```python
from build123d import *

# Parameters (mm, degrees)
SKETCH_1_R          = 7.65
EXTRUDE_1_DEPTH     = 3
SKETCH_2_R          = 5
CUT_EXTRUDE_1_DEPTH = 366.286189172
FILLET_1_R          = 20
SKETCH_3_R          = 1.65
CUT_EXTRUDE_2_DEPTH = 366.286189172
FILLET_2_R          = 40
FILLET_3_R          = 80
SKETCH_4_W          = 105
SKETCH_4_H          = 60
CUT_EXTRUDE_3_DEPTH = 366.286189172
FILLET_4_R          = 5
CUT_EXTRUDE_4_DEPTH = 269.344927286
FILLET_5_R          = 2
FILLET_6_R          = 8
EXTRUDE_START       = -3
EXTRUDE_2_DEPTH     = 3
SKETCH_7_R          = 1.65
CUT_EXTRUDE_5_DEPTH = 3


with BuildPart() as part:
    # 草图1 → 凸台-拉伸1 (new body)
    with BuildSketch(Plane.XY):
        with BuildLine():
            Line((106.954174428, -60), (20.632339437, 21.778580517))
            ThreePointArc((20.632339437, 21.778580517), (-21.778580517, 20.632339437), (-20.632339437, -21.778580517))
            Line((-20.632339437, -21.778580517), (83.045825572, -120))
            Line((83.045825572, -120), (345, -120))
            Line((345, -120), (345, -60))
            Line((345, -60), (106.954174428, -60))
        make_face()
        Circle(SKETCH_1_R, mode=Mode.SUBTRACT)
    extrude(amount=EXTRUDE_1_DEPTH)

    # 草图2 → 切除-拉伸1 (cut, through all)
    with BuildSketch(Plane.XY.offset(3)):
        with Locations((305, -90)):
            Circle(SKETCH_2_R)
        with Locations((278, -90)):
            Circle(SKETCH_2_R)
        with Locations((332, -90)):
            Circle(SKETCH_2_R)
    extrude(amount=-CUT_EXTRUDE_1_DEPTH, mode=Mode.SUBTRACT)

    # 圆角1
    fillet_1_edges = [part.edges().sort_by_distance(p)[0] for p in [
        (345, -60, 1.5),
        (345, -120, 1.5),
    ]]
    fillet(fillet_1_edges, radius=FILLET_1_R)

    # 草图3 → 切除-拉伸2 (cut, through all)
    with BuildSketch(Plane.XY.offset(3)):
        with Locations((216.4, -115.5)):
            Circle(SKETCH_3_R)
        with Locations((216.5, -64.5)):
            Circle(SKETCH_3_R)
        with Locations((191.5, -64.5)):
            Circle(SKETCH_3_R)
        with Locations((191.4, -115.5)):
            Circle(SKETCH_3_R)
        with Locations((14.114048497, -48.497460089)):
            Circle(SKETCH_3_R)
        with Locations((49.18902554, -11.473873209)):
            Circle(SKETCH_3_R)
        with Locations((67.385880926, -28.616640024)):
            Circle(SKETCH_3_R)
        with Locations((32.310903883, -65.640226903)):
            Circle(SKETCH_3_R)
        with BuildLine():
            Line((222.8, -113.85), (235, -113.85))
            ThreePointArc((235, -113.85), (236.65, -115.5), (235, -117.15))
            Line((235, -117.15), (222.8, -117.15))
            ThreePointArc((222.8, -117.15), (221.15, -115.5), (222.8, -113.85))
        make_face()
        with BuildLine():
            Line((222.8, -66.15), (235, -66.15))
            ThreePointArc((235, -66.15), (236.65, -64.5), (235, -62.85))
            Line((235, -62.85), (222.8, -62.85))
            ThreePointArc((222.8, -62.85), (221.15, -64.5), (222.8, -66.15))
        make_face()
        with BuildLine():
            Line((36.821084288, 2.51599917), (45.677707032, -5.874485534))
            ThreePointArc((45.677707032, -5.874485534), (45.740750291, -8.207086132), (43.408149694, -8.270129391))
            Line((43.408149694, -8.270129391), (34.55152695, 0.120355313))
            ThreePointArc((34.55152695, 0.120355313), (34.488483691, 2.452955911), (36.821084288, 2.51599917))
        make_face()
        with BuildLine():
            Line((19.942962631, -51.650354523), (28.799585375, -60.040839228))
            ThreePointArc((28.799585375, -60.040839228), (28.862628634, -62.373439825), (26.530028037, -62.436483085))
            Line((26.530028037, -62.436483085), (17.673405293, -54.04599838))
            ThreePointArc((17.673405293, -54.04599838), (17.610362034, -51.713397783), (19.942962631, -51.650354523))
        make_face()
        with BuildLine():
            Line((197.8, -113.85), (210, -113.85))
            ThreePointArc((210, -113.85), (211.65, -115.5), (210, -117.15))
            Line((210, -117.15), (197.8, -117.15))
            ThreePointArc((197.8, -117.15), (196.15, -115.5), (197.8, -113.85))
        make_face()
        with BuildLine():
            Line((197.8, -66.15), (210, -66.15))
            ThreePointArc((210, -66.15), (211.65, -64.5), (210, -62.85))
            Line((210, -62.85), (197.8, -62.85))
            ThreePointArc((197.8, -62.85), (196.15, -64.5), (197.8, -66.15))
        make_face()
        with BuildLine():
            Line((172.8, -113.85), (185, -113.85))
            ThreePointArc((185, -113.85), (186.65, -115.5), (185, -117.15))
            Line((185, -117.15), (172.8, -117.15))
            ThreePointArc((172.8, -117.15), (171.15, -115.5), (172.8, -113.85))
        make_face()
        with BuildLine():
            Line((172.8, -66.15), (185, -66.15))
            ThreePointArc((185, -66.15), (186.65, -64.5), (185, -62.85))
            Line((185, -62.85), (172.8, -62.85))
            ThreePointArc((172.8, -62.85), (171.15, -64.5), (172.8, -66.15))
        make_face()
        with BuildLine():
            Line((1.746107245, -34.507587709), (10.602729989, -42.898072413))
            ThreePointArc((10.602729989, -42.898072413), (10.665773248, -45.230673011), (8.333172651, -45.29371627))
            Line((8.333172651, -45.29371627), (-0.523450093, -36.903231566))
            ThreePointArc((-0.523450093, -36.903231566), (-0.586493353, -34.570630968), (1.746107245, -34.507587709))
        make_face()
        with BuildLine():
            Line((55.017939675, -14.626767644), (63.874562418, -23.017252349))
            ThreePointArc((63.874562418, -23.017252349), (63.937605678, -25.349852946), (61.60500508, -25.412896206))
            Line((61.60500508, -25.412896206), (52.748382337, -17.022411501))
            ThreePointArc((52.748382337, -17.022411501), (52.685339077, -14.689810904), (55.017939675, -14.626767644))
        make_face()
        with BuildLine():
            Line((38.139818017, -68.793121338), (46.996440761, -77.183606042))
            ThreePointArc((46.996440761, -77.183606042), (47.05948402, -79.51620664), (44.726883423, -79.579249899))
            Line((44.726883423, -79.579249899), (35.870260679, -71.188765195))
            ThreePointArc((35.870260679, -71.188765195), (35.80721742, -68.856164597), (38.139818017, -68.793121338))
        make_face()
        with BuildLine():
            Line((73.214795061, -31.769534459), (82.071417805, -40.160019163))
            ThreePointArc((82.071417805, -40.160019163), (82.134461064, -42.492619761), (79.801860466, -42.55566302))
            Line((79.801860466, -42.55566302), (70.945237723, -34.165178315))
            ThreePointArc((70.945237723, -34.165178315), (70.882194463, -31.832577718), (73.214795061, -31.769534459))
        make_face()
    extrude(amount=-CUT_EXTRUDE_2_DEPTH, mode=Mode.SUBTRACT)

    # 圆角2
    fillet_2_edges = [part.edges().sort_by_distance(p)[0] for p in [
        (106.954174428, -60, 1.5),
    ]]
    fillet(fillet_2_edges, radius=FILLET_2_R)

    # 圆角3
    fillet_3_edges = [part.edges().sort_by_distance(p)[0] for p in [
        (83.045825572, -120, 1.5),
    ]]
    fillet(fillet_3_edges, radius=FILLET_3_R)

    # 草图4 → 切除-拉伸3 (cut, through all)
    with BuildSketch(Plane.XY.offset(3)):
        with Locations((292.5, -90)):
            Rectangle(SKETCH_4_W, SKETCH_4_H)
    extrude(amount=-CUT_EXTRUDE_3_DEPTH, mode=Mode.SUBTRACT)

    # 圆角4
    fillet_4_edges = [part.edges().sort_by_distance(p)[0] for p in [
        (240, -120, 1.5),
        (240, -60, 1.5),
    ]]
    fillet(fillet_4_edges, radius=FILLET_4_R)

    # 草图5 → 切除-拉伸4 (cut, through all)
    with BuildSketch(Plane.XY.offset(3)):
        Polygon((170.8, -107.073879127), (170.8, -72.926120873), (196.643481613, -90), align=None)
        Polygon((107.673788457, -69), (162.8, -69), (162.8, -112), align=None)
        Polygon((182.624652559, -71.15), (203.9, -85.205873586), (225.175347441, -71.15), align=None)
        Polygon((211.156518387, -90), (237, -72.926120873), (237, -107.073879127), align=None)
        Polygon((182.624652559, -108.85), (203.9, -94.794126414), (225.175347441, -108.85), align=None)
        Polygon((104.589547434, -76.740160666), (149.792834925, -112), (90.539471777, -112), align=None)
        Polygon((83.107750181, -109.038663458), (97.619712786, -72.619680215), (53.254218477, -80.756370264), align=None)
        Polygon((60.248478543, -73.373540194), (82.827238337, -49.540404857), (100.242066861, -66.038663458), align=None)
        Polygon((12.415001138, -37.631100304), (37.481546744, -42.016378913), (43.304983555, -66.895294173), align=None)
        Polygon((38.334111759, -10.557272346), (44.066420967, -35.046871816), (68.740714664, -39.36352773), align=None)
        Polygon((46.048599826, -43.515146043), (73.041613266, -48.237451473), (52.282913666, -70.149412161), align=None)
    extrude(amount=-CUT_EXTRUDE_4_DEPTH, mode=Mode.SUBTRACT)

    # 圆角5
    fillet_5_edges = [part.edges().sort_by_distance(p)[0] for p in [
        (53.254218477, -80.756370264, 1.5),
        (97.619712786, -72.619680215, 1.5),
        (104.589547434, -76.740160666, 1.5),
        (149.792834925, -112, 1.5),
        (100.242066861, -66.038663458, 1.5),
        (60.248478543, -73.373540194, 1.5),
        (82.827238337, -49.540404857, 1.5),
        (43.304983555, -66.895294173, 1.5),
        (12.415001138, -37.631100304, 1.5),
        (37.481546744, -42.016378913, 1.5),
        (237, -107.073879127, 1.5),
        (211.156518387, -90, 1.5),
        (237, -72.926120873, 1.5),
        (182.624652559, -71.15, 1.5),
        (225.175347441, -71.15, 1.5),
        (203.9, -85.205873586, 1.5),
        (225.175347441, -108.85, 1.5),
        (182.624652559, -108.85, 1.5),
        (203.9, -94.794126414, 1.5),
        (162.8, -112, 1.5),
        (107.673788457, -69, 1.5),
        (162.8, -69, 1.5),
        (38.334111759, -10.557272346, 1.5),
        (68.740714664, -39.36352773, 1.5),
        (44.066420967, -35.046871816, 1.5),
        (52.282913666, -70.149412161, 1.5),
        (46.048599826, -43.515146043, 1.5),
        (73.041613266, -48.237451473, 1.5),
        (196.643481613, -90, 1.5),
        (170.8, -107.073879127, 1.5),
        (170.8, -72.926120873, 1.5),
    ]]
    fillet(fillet_5_edges, radius=FILLET_5_R)

    # 圆角6
    fillet_6_edges = [part.edges().sort_by_distance(p)[0] for p in [
        (83.107750181, -109.038663458, 1.5),
        (90.539471777, -112, 1.5),
    ]]
    fillet(fillet_6_edges, radius=FILLET_6_R)

    # 草图6 → 凸台-拉伸2 (add)
    with BuildSketch(Plane.XY.offset(3).offset(EXTRUDE_START)):
        with BuildLine():
            Line((-27.891866276, -14.901134038), (-20.632339437, -21.778580517))
            ThreePointArc((-20.632339437, -21.778580517), (-21.778580517, 20.632339437), (20.632339437, 21.778580517))
            Line((20.632339437, 21.778580517), (13.372812598, 28.656026996))
            ThreePointArc((13.372812598, 28.656026996), (-29.038107356, 27.509785916), (-27.891866276, -14.901134038))
        make_face()
    extrude(amount=EXTRUDE_2_DEPTH)

    # 草图7 → 切除-拉伸5 (cut)
    with BuildSketch(Plane.XY.offset(3)):
        with Locations((-21.778580517, 20.632339437)):
            Circle(SKETCH_7_R)
        with Locations((21.778580517, -20.632339437)):
            Circle(SKETCH_7_R)
    extrude(amount=-CUT_EXTRUDE_5_DEPTH, mode=Mode.SUBTRACT)


solid = part.part
```
Model file for the job. Use its own axes, mm. A direction names the side the tool comes from. Coordinates: 2 decimals unless noted, no trailing zeros. Order: outer loops, then holes, each group sorted by start corner. A loop starts at its lowest first (then second) coordinate and runs counter-clockwise, first axis right, second up. Notation, with made-up numbers: (-24.75, 38) -> (-6.75, 38) arc R35 cw to (-6.75, 74) -> close; hole circle Ø7 at (29.25, 49.5). An arc over 180 degrees is marked (long way). Answer as a JSON object with one key per item and string values. Group by question number.
1) Cut at A-A, the plane z = 1.5. Count the separate pieces of the cut face and the enclosed holes in it, then the cut area to 3 significant figures.
2) Cut at B-B, the plane y = 25.5. Write the cut outline in (x, z), then the cut area to 3 significant figures.
3) Flat gauge pins, fed straight in: pin 1 (0.9 mm diameter, centred on y = -96.5, z = 1.5, fed in from -X); pin 2 (2.5 mm diameter, centred on x = 191.5, y = -64.5, fed in from +Z); pin 3 (1.5 mm diameter, centred on x = 227, z = 1.5, fed in from +Y); pin 4 (1.5 mm diameter, centred on x = 115, z = 1.5, fed in from +Y). Where does each tip first touch, or does it go through?
4) Drill centre lines: L1, parallel to X at y = 1.5, z = 1.45; L2, parallel to Y at x = 203.5, z = 1.2; L3, parallel to Y at x = 75, z = 2.25. Where is each one in solid material? Low to high.
5) Pull direction Y, two halves, no side cores. Call faces 1 (the face through (70, -41, 3)), 2 (the face through (6.11, -38.64, 1.52)), 3 (the face through (84.92, -114.16, 1.52)): +Y half, -Y half, draft (parallel to the pull), parting line (faces both ways), or undercut.
6) Which spindle directions (+Z, -Z, +X, -X, +Y, -Y) get a long thin tool onto all of the face, cutting with end or side? Do faces 4 (the face through (54.952, -10.735, 1.479)), 5 (the face through (212.21, -100.284, 1.521)). Say none if no direction does.
Check values:
{
 "1": {"separate pieces": "1", "enclosed holes": "34", "area": "12,000 mm²"},
 "2": {"outline": "(-30.78, 0) -> (16.7, 0) -> (16.7, 3) -> (-30.78, 3) -> close", "area": "142 mm²"},
 "3": {"pin 1": "stops at x = 57.77", "pin 2": "passes through", "pin 3": "stops at y = -60", "pin 4": "stops at y = -59.06"},
 "4": {"L1": "x = -36.77 to -7.5, 7.5 to 34.05, 37.89 to 42.04", "L2": "y = -120 to -117.15, -113.85 to -108.85, -95.23 to -84.77, -71.15 to -66.15, -62.85 to -60", "L3": "y = -109.33 to -101.33, -76.77 to -70.67, -57.8 to -38.01, -33.46 to -29.73"},
 "5": {"face 1": "draft", "face 2": "undercut", "face 3": "-Y half"},
 "6": {"face 4": "+Z, -Z, +X, +Y", "face 5": "+Z, -Z"}
}
